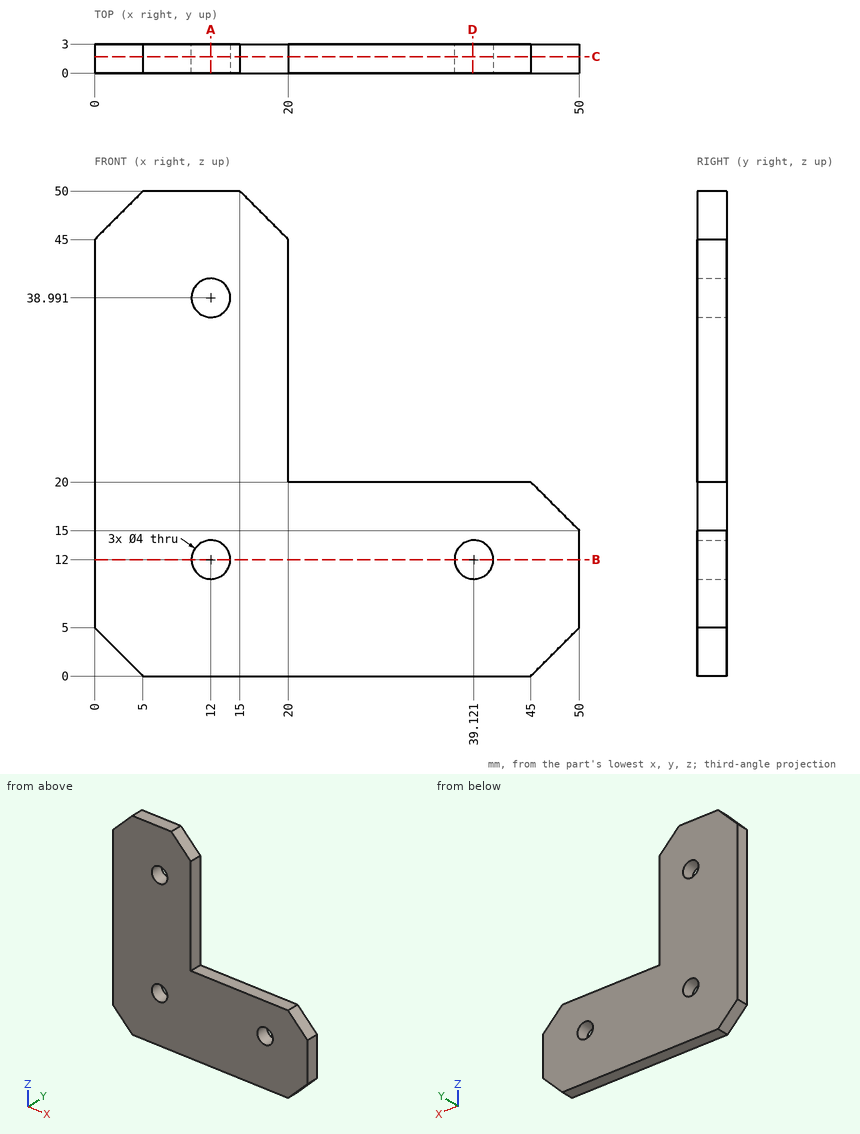
For this review, use the dimensioned drawing (mm, ordinates from the lowest corner) and the shaded views. Give positions to 0.01 mm unless a question says otherwise; leave off trailing zeros. Write each loop counter-clockwise with the first axis right and the second up, starting at its lowest first coordinate (ties: lowest second). Pieces come first, ordered by that corner, then holes. Notation, with made-up numbers: M 71.5,76.25 L 106.5,76.25 A16 ccw 106.5,103.25 Z; hole C -17.5,85.5 d2. An arc over 180 degrees is marked long. Answer as a JSON object with one key per item and string values. Group by question number.
Item 1: For probe 1 along Z at (x, y) = (12, 0.7); probe 2 along Z at (x, y) = (37, 0.4), list the stretches that pass through material, from the lowest coordinate up. Write a range as [from, to].
Item 2: Consider section A-A on x = 12. Write out the cut boundary in (y, z), plus the area to 3 significant figures.
Item 3: Consider section D-D on x = 39. Write out the cut boundary in (y, z).
Item 4: For pin 1 Ø1.5 at (y, z) = (2, 32) entering from +X; pin 2 Ø3 at (x, z) = (12, 38.99) entering from -Y (1 decimal), all flat-tipped, find the tip position at first contact; note any pin that passes through.
Item 5: Consider section B-B on z = 12. Write out the cut boundary in (x, y), plus the area to 3 significant figures.
Item 6: Consider section C-C on y = 1.7. Write out the cut boundary in (x, z).
Check result:
{
 "1": {"probe 1": "z = [0, 10], [14, 36.99], [40.99, 50]", "probe 2": "z = [0, 20]"},
 "2": {"outline": "M 0,0 L 3,0 L 3,10 L 0,10 Z; M 0,14 L 3,14 L 3,36.99 L 0,36.99 Z; M 0,40.99 L 3,40.99 L 3,50 L 0,50 Z", "area": "126 mm^2"},
 "3": {"outline": "M 0,0 L 3,0 L 3,10 L 0,10 Z; M 0,14 L 3,14 L 3,20 L 0,20 Z"},
 "4": {"pin 1": "stops at x = 20", "pin 2": "passes through"},
 "5": {"outline": "M 0,0 L 10,0 L 10,3 L 0,3 Z; M 14,0 L 37.12,0 L 37.12,3 L 14,3 Z; M 41.12,0 L 50,0 L 50,3 L 41.12,3 Z", "area": "126 mm^2"},
 "6": {"outline": "M 0,5 L 5,0 L 45,0 L 50,5 L 50,15 L 45,20 L 20,20 L 20,45 L 15,50 L 5,50 L 0,45 Z; hole C 12,12 d4; hole C 12,38.99 d4; hole C 39.12,12 d4"}
}
